```python
from build123d import *

# Parameters (mm, degrees)
CYLINDER_R               = 6
CYLINDER_DEPTH           = 60
CYLINDER001_R            = 2.5
CYLINDER001_DEPTH        = 40
ARRAY001_COUNT           = 4
ARRAY001_PLACEMENT_ANGLE = 45
BOX007_W                 = 40
BOX007_H                 = 40
BOX007_DEPTH             = 10
FILLET001_R              = 5
CYLINDER003_R            = 70
CYLINDER003_DEPTH        = 20
CYLINDER004_R            = 4
CYLINDER004_DEPTH        = 60
CYLINDER005_R            = 2
CYLINDER005_DEPTH        = 40
BODY004_PLACEMENT_ANGLE  = 90
BODY003_PLACEMENT_ANGLE  = 90
BOX005_W                 = 24
BOX005_H                 = 24
BOX005_DEPTH             = 50
CUT002_PLACEMENT_ANGLE   = 15
BOX006_W                 = 120
BOX006_H                 = 100
BOX006_DEPTH             = 5
FILLET_R                 = 10


with BuildPart() as cone001:
    # Cone001 → Cone001 (revolve)
    with BuildSketch(Plane.XZ):
        Polygon((0, 0), (2.5, 0), (6, 4), (0, 4), align=None)
    revolve(axis=Axis((0, 0, 0), (0, 0, 1)))


with BuildPart() as cylinder:
    # Cylinder → Cylinder (new body)
    with BuildSketch(Plane.XY.offset(4)):
        Circle(CYLINDER_R)
    extrude(amount=CYLINDER_DEPTH)


with BuildPart() as screw_hole_clone:
    # Cylinder001 → Cylinder001 (new body)
    with BuildSketch(Plane.XY.offset(-40)):
        Circle(CYLINDER001_R)
    extrude(amount=CYLINDER001_DEPTH)

    # Fusion002: union Cone001, Cylinder
    add(cone001.part)
    add(cylinder.part)


with BuildPart() as screw_hole_clone_1:
    # Fusion002 placement: moved
    add(screw_hole_clone.part.moved(Location((0, 0, 5))))


with BuildPart() as screw_hole_clone_2:
    # Body001 placement: moved
    add(screw_hole_clone_1.part.moved(Location((0, 0, -5))))


with BuildPart() as array001:
    # Body002 base: copy of screw hole clone
    add(screw_hole_clone_2.part)


with BuildPart() as array001_1:
    # Body002 placement: moved
    add(array001.part.moved(Location((0, 53, 0))))

    # Array001: Array001 ×4 about axis
    array001_axis = Axis((0, 0, 0), (0, 0, 1))


with BuildPart() as array001_2:
    add(array001_1.part)
    for i in range(1, ARRAY001_COUNT):
        add(array001_1.part.rotate(array001_axis, i * 360 / ARRAY001_COUNT))


with BuildPart() as array001_3:
    # Array001 placement: moved
    add(array001_2.part.rotate(Axis((0, 0, 0), (0, 0, 1)), ARRAY001_PLACEMENT_ANGLE))


with BuildPart() as central_hole_cube_fillet:
    # Box007 → Box007 (new body)
    with BuildSketch(Plane(origin=(-20, -20, 0), x_dir=(1, 0, 0), z_dir=(0, 0, 1))):
        with Locations((20, 20)):
            Rectangle(BOX007_W, BOX007_H)
    extrude(amount=BOX007_DEPTH)

    # Fillet001
    fillet001_edges = [central_hole_cube_fillet.edges().sort_by_distance(p)[0] for p in [
        (-20, -20, 5),
        (-20, 20, 5),
        (20, -20, 5),
        (20, 20, 5),
    ]]
    fillet(fillet001_edges, radius=FILLET001_R)


with BuildPart() as extraction_fusion:
    # Cylinder003 → Cylinder003 (new body)
    with BuildSketch(Plane.XY.offset(-20)):
        Circle(CYLINDER003_R)
    extrude(amount=CYLINDER003_DEPTH)

    # Fusion006: union screw hole clone, Array001, central hole cube fillet
    add(screw_hole_clone_2.part)
    add(array001_3.part)
    add(central_hole_cube_fillet.part)


with BuildPart() as cone002:
    # Cone002 → Cone002 (revolve)
    with BuildSketch(Plane.XZ):
        Polygon((0, 0), (2, 0), (4, 4), (0, 4), align=None)
    revolve(axis=Axis((0, 0, 0), (0, 0, 1)))


with BuildPart() as cylinder004:
    # Cylinder004 → Cylinder004 (new body)
    with BuildSketch(Plane.XY.offset(4)):
        Circle(CYLINDER004_R)
    extrude(amount=CYLINDER004_DEPTH)


with BuildPart() as m3_screw_hole_fusion:
    # Cylinder005 → Cylinder005 (new body)
    with BuildSketch(Plane.XY.offset(-40)):
        Circle(CYLINDER005_R)
    extrude(amount=CYLINDER005_DEPTH)

    # Fusion007: union Cone002, Cylinder004
    add(cone002.part)
    add(cylinder004.part)


with BuildPart() as m3_screw_hole_fusion_1:
    # Fusion007 placement: moved
    add(m3_screw_hole_fusion.part.moved(Location((0, 0, 5))))


with BuildPart() as m3_screw_hole_fusion_clone001:
    # Body004 base: copy of m3 screw hole fusion
    add(m3_screw_hole_fusion_1.part)


with BuildPart() as m3_screw_hole_fusion_clone001_1:
    # Body004 placement: moved
    add(m3_screw_hole_fusion_clone001.part.moved(Location((12, 26, 37))).rotate(Axis((12, 26, 37), (1, 0, 0)), BODY004_PLACEMENT_ANGLE))


with BuildPart() as m3_hole_fusion:
    # Body003 base: copy of m3 screw hole fusion
    add(m3_screw_hole_fusion_1.part)


with BuildPart() as m3_hole_fusion_1:
    # Body003 placement: moved
    add(m3_hole_fusion.part.moved(Location((-2, 12, 22))).rotate(Axis((-2, 12, 22), (0, 1, 0)), BODY003_PLACEMENT_ANGLE))

    # Fusion008: union m3 screw hole fusion clone001
    add(m3_screw_hole_fusion_clone001_1.part)


with BuildPart() as cube_cut:
    # Box005 → Box005 (new body)
    with BuildSketch(Plane.XY):
        with Locations((12, 12)):
            Rectangle(BOX005_W, BOX005_H)
    extrude(amount=BOX005_DEPTH)

    # Cut002: cut m3 hole fusion
    add(m3_hole_fusion_1.part, mode=Mode.SUBTRACT)


with BuildPart() as cube_cut_1:
    # Cut002 placement: moved
    add(cube_cut.part.moved(Location((28.9778, -7.23543, 0))).rotate(Axis((28.9778, -7.23543, 0), (0, 1, 0)), CUT002_PLACEMENT_ANGLE))


with BuildPart() as base_cube_fillet:
    # Box006 → Box006 (new body)
    with BuildSketch(Plane(origin=(-60, -50, 0), x_dir=(1, 0, 0), z_dir=(0, 0, 1))):
        with Locations((60, 50)):
            Rectangle(BOX006_W, BOX006_H)
    extrude(amount=BOX006_DEPTH)

    # Fillet
    fillet_edges = [base_cube_fillet.edges().sort_by_distance(p)[0] for p in [
        (-60, -50, 2.5),
        (-60, 50, 2.5),
        (60, -50, 2.5),
        (60, 50, 2.5),
    ]]
    fillet(fillet_edges, radius=FILLET_R)


with BuildPart() as stand_cut_v2:
    # Part__Mirroring001: instance of cube cut
    add(cube_cut_1.part.mirror(Plane(origin=(0, 7, 0), x_dir=(0, -1, 0), z_dir=(1, 0, 0))))

    # Fusion005: union cube cut, base cube fillet
    add(cube_cut_1.part)
    add(base_cube_fillet.part)

    # Cut001: cut extraction fusion
    add(extraction_fusion.part, mode=Mode.SUBTRACT)


solid = stand_cut_v2.part
```
Model file for the job. Use its own axes, mm. A direction names the side the tool comes from. Round coordinates to 2 decimals unless told otherwise and drop trailing zeros. Write each loop counter-clockwise with the first axis right and the second up, starting at its lowest first coordinate (ties: lowest second). Pieces come first, ordered by that corner, then holes. Notation, with made-up numbers: (61, -8) - (74, -8) arc R14 ccw to (74, 12) - close; hole circle Ø2 at (22.25, -14). An arc over 180 degrees is marked (long way). One line per item, written item: value.
(1) 3-axis set-ups, long thin cutter, end or side, ignore diameter. For faces 4 (the conical face through (-37.66, 5.47, 18.13)), 5 (the cylindrical face through (19, 18, 3)), 6 (the cylindrical face through (48, 1.38, 36.01)): which of +Z, -Z, +X, -X, +Y, -Y reach the whole face in a straight line?
Values follow:
face 4: none
face 5: +Z, -Z
face 6: -Y
(2) Wall check: probe 1 along Y at (x, z) = (0.5, 2.5); probe 2 along X at (y, z) = (-7.5, 2.5); probe 3 along Z at (x, y) = (-4, -35). Give the ranges that are in metal, low to high.
Values follow:
probe 1: y = -50 to -20, 20 to 50
probe 2: x = -60 to -20, 20 to 60
probe 3: z = 0 to 5
(3) Cut at B-B, the plane x = 26. Give the cut face in (y, z), plus the area to 3 significant figures.
Values follow:
outline: (-50, 0) - (50, 0) - (50, 5) - (-50, 5) - close
area: 500 mm²
(4) Cut at A-A, the plane z = 6.5. Give the cut face in (x, y), plus the area to 3 significant figures.
Values follow:
outline: (-55.57, -7.24) - (-30.72, -7.24) - (-30.72, 16.76) - (-55.57, 16.76) - close; (30.72, -7.24) - (55.57, -7.24) - (55.57, 16.76) - (30.72, 16.76) - close
area: 1,190 mm²
(5) Drop flat-ended pins along their axis: P1, Ø4, axis at y = 3, z = 3.5, coming from the +X side; P2, Ø10.5, axis at x = 41.5, z = 28.5, coming from the +Y side; P3, Ø10, axis at y = 1, z = 7, coming from the -X side; P4, Ø3, axis at x = 50.15, z = 32.63, coming from the -Y side. Give the stop position or say it passes through.
Values follow:
P1: stops at x = 60
P2: stops at y = 16.76
P3: stops at x = -60
P4: passes through
(6) Two-plate mould, pull along Y, no slides. Class faces 1 (the cylindrical face through (-19, 18, 3)), 2 (the flat face through (-53.348, 4.933, 45.234)), 3 (the flat face through (47, 16.765, 23)): pulls with the +Y half, pulls with the -Y half, needs draft (parallel to the pull), parting line crosses it, or undercut.
Values follow:
face 1: undercut
face 2: needs draft
face 3: pulls with the +Y half
